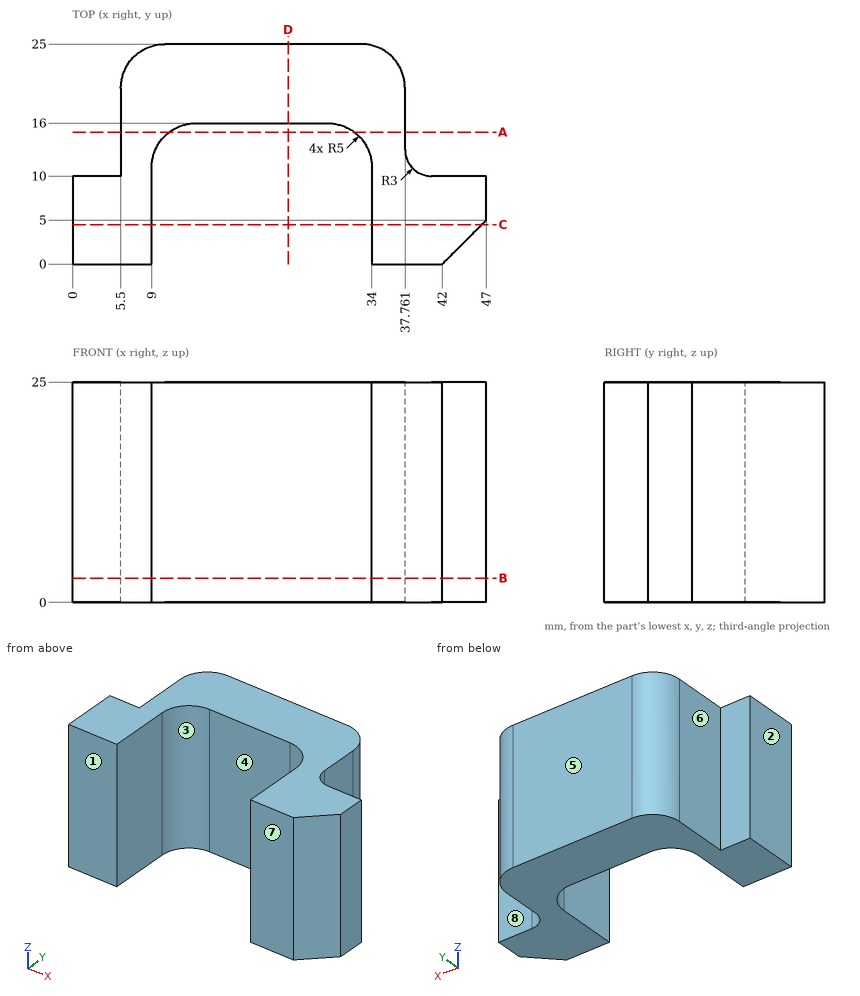
Verification items for this drawing (mm, ordinates from the low corner). A direction names the side the tool comes from. Coordinates: 2 decimals unless noted, no trailing zeros. Write each loop counter-clockwise with the first axis right and the second up, starting at its lowest first coordinate (ties: lowest second). Pieces come first, ordered by that corner, then holes. Notation, with made-up numbers: (83, 72.5) -> (125, 72.5) arc R30 cw to (125, 97.5) -> close; hole circle Ø1 at (-18, 69.5). An arc over 180 degrees is marked (long way). One line per item, written item: value. Start each with the question number.
Q1. Cross-section at C-C on y = 4.5. Enter the section's corners in (x, z).
Q2. Cross-section at B-B on z = 2.75. Enter the section's corners in (x, y), and give its area (3 significant figures).
Q3. Mould release check, pull along X, two halves, no side actions. Record for the marked faces 1, 2 and 3: pulls with the +X half, pulls with the -X half, needs draft (parallel to the pull), parting line crosses it, or undercut.
Q4. Cross-section at A-A on y = 15. Enter the section's corners in (x, z).
Q5. Thickness scan on L1, parallel to X at y = 8.75, z = 1.75; L2, parallel to X at y = 3.75, z = 9.5; L3, parallel to Y at x = 25, z = 8.5. Record the ranges inside material, lowest first. Write a range as from..to.
Q6. Access from +Z, -Z, +X, -X, +Y, -Y to the whole of each face (thin tool, end or side, straight path). Record for the marked faces 4, 5, 6, 7 and 8.
Q7. Cross-section at D-D on x = 24.5. Enter the section's corners in (y, z).
Q8. Go/stop test with flat-tipped pins: P1, Ø2, axis at y = 15.5, z = 12, coming from the +X side; P2, Ø1.9, axis at x = 43.5, z = 13, coming from the +Y side; P3, Ø7.5, axis at x = 23.5, z = 14.5, coming from the -Y side. Record where each tip stops, or that it passes through.
Checked values:
1. outline: (0, 0) -> (9, 0) -> (9, 25) -> (0, 25) -> close; (34, 0) -> (46.5, 0) -> (46.5, 25) -> (34, 25) -> close
2. outline: (0, 0) -> (9, 0) -> (9, 11) arc R5 cw to (14, 16) -> (29, 16) arc R5 cw to (34, 11) -> (34, 0) -> (42, 0) -> (47, 5) -> (47, 10) -> (40.76, 10) arc R3 cw to (37.76, 13) -> (37.76, 20) arc R5 ccw to (32.76, 25) -> (10.5, 25) arc R5 ccw to (5.5, 20) -> (5.5, 10) -> (0, 10) -> close
2. area: 543 mm²
3. face 1: needs draft
3. face 2: pulls with the -X half
3. face 3: undercut
4. outline: (5.5, 0) -> (11, 0) -> (11, 25) -> (5.5, 25) -> close; (32, 0) -> (37.76, 0) -> (37.76, 25) -> (32, 25) -> close
5. L1: x = 0..9, 34..47
5. L2: x = 0..9, 34..45.75
5. L3: y = 16..25
6. face 4: +Z, -Z, -Y
6. face 5: +Z, -Z, +X, -X, +Y
6. face 6: +Z, -Z, -X, +Y
6. face 7: +Z, -Z, +X, -X, -Y
6. face 8: +Z, -Z, +X, +Y
7. outline: (16, 0) -> (25, 0) -> (25, 25) -> (16, 25) -> close
8. P1: stops at x = 37.76
8. P2: stops at y = 10
8. P3: stops at y = 16
